from build123d import *

# Parameters (mm, degrees)
SKETCH1_R           = 14.45
BOSS_EXTRUDE1_DEPTH = 14
BOSS_EXTRUDE2_START = 7.6
SKETCH2_W           = 35.45
SKETCH2_H           = 36.25
BOSS_EXTRUDE2_DEPTH = 7.6
FILLET1_R           = 10
CUT_EXTRUDE1_REACH  = 44.204
SKETCH3_R           = 2.3
CHAMFER1_SIZE       = 0.5
CHAMFER2_SIZE       = 0.2
CHAMFER2_SIZE2      = 5.727250657
CHAMFER3_SIZE       = 0.5


with BuildPart() as part:
    # Sketch1 → Boss-Extrude1 (new body)
    with BuildSketch(Plane.XY):
        Circle(SKETCH1_R)
        with BuildLine():
            Line((-8.510102807, -10.125), (8.510102807, -10.125))
            ThreePointArc((8.510102807, -10.125), (9.652007563, -9.652007563), (10.125, -8.510102807))
            Line((10.125, -8.510102807), (10.125, 8.510102807))
            ThreePointArc((10.125, 8.510102807), (9.652007563, 9.652007563), (8.510102807, 10.125))
            Line((8.510102807, 10.125), (-8.510102807, 10.125))
            ThreePointArc((-8.510102807, 10.125), (-9.652007563, 9.652007563), (-10.125, 8.510102807))
            Line((-10.125, 8.510102807), (-10.125, -8.510102807))
            ThreePointArc((-10.125, -8.510102807), (-9.652007563, -9.652007563), (-8.510102807, -10.125))
        make_face(mode=Mode.SUBTRACT)
    extrude(amount=BOSS_EXTRUDE1_DEPTH)

    # Sketch2 → Boss-Extrude2 (add)
    with BuildSketch(Plane(origin=(0, 0, 0), x_dir=(-1, 0, 0), z_dir=(0, 0, -1)).offset(BOSS_EXTRUDE2_START)):
        with Locations((-0.4, 0)):
            Rectangle(SKETCH2_W, SKETCH2_H)
        with BuildLine():
            Line((8.510102807, -10.125), (-8.510102807, -10.125))
            ThreePointArc((-8.510102807, -10.125), (-9.652007563, -9.652007563), (-10.125, -8.510102807))
            Line((-10.125, -8.510102807), (-10.125, 8.510102807))
            ThreePointArc((-10.125, 8.510102807), (-9.652007563, 9.652007563), (-8.510102807, 10.125))
            Line((-8.510102807, 10.125), (8.510102807, 10.125))
            ThreePointArc((8.510102807, 10.125), (9.652007563, 9.652007563), (10.125, 8.510102807))
            Line((10.125, 8.510102807), (10.125, -8.510102807))
            ThreePointArc((10.125, -8.510102807), (9.652007563, -9.652007563), (8.510102807, -10.125))
        make_face(mode=Mode.SUBTRACT)
    extrude(amount=-BOSS_EXTRUDE2_DEPTH)

    # Fillet1
    fillet1_edges = [part.edges().sort_by_distance(p)[0] for p in [
        (18.125, 18.125, -3.8),
        (18.125, -18.125, -3.8),
        (-17.325, -18.125, -3.8),
        (-17.325, 18.125, -3.8),
    ]]
    fillet(fillet1_edges, radius=FILLET1_R)

    # Sketch3 → Cut-Extrude1 (cut, up to next)
    with BuildSketch(Plane.ZY.offset(17.325), mode=Mode.PRIVATE) as cut_extrude1_sk1:
        with Locations(Location((-3.8, 0, 0), (0, 0, 270))):
            Circle(SKETCH3_R)
    cut_extrude1_tool1 = extrude(cut_extrude1_sk1.sketch, amount=-CUT_EXTRUDE1_REACH, mode=Mode.PRIVATE) & part.part
    add(cut_extrude1_tool1.solids().sort_by_distance((-17.325, 0, -3.8))[0], mode=Mode.SUBTRACT)

    # Chamfer1
    chamfer1_edges = [part.edges().sort_by_distance(p)[0] for p in [
        (-9.652007563, 9.652007563, -7.6),
        (0, 10.125, -7.6),
        (9.652007563, 9.652007563, -7.6),
        (10.125, 0, -7.6),
        (9.652007563, -9.652007563, -7.6),
        (0, -10.125, -7.6),
        (-9.652007563, -9.652007563, -7.6),
        (-10.125, 0, -7.6),
        (0.4, 18.125, 0),
        (0.4, 18.125, -7.6),
        (18.125, 0, 0),
        (-17.325, 0, 0),
        (0.4, -18.125, 0),
        (-14.396067812, -15.196067812, 0),
        (15.196067812, -15.196067812, 0),
        (15.196067812, 15.196067812, 0),
        (-14.396067812, 15.196067812, 0),
        (-17.325, 0, -7.6),
        (18.125, 0, -7.6),
        (0.4, -18.125, -7.6),
        (-14.396067812, -15.196067812, -7.6),
        (15.196067812, -15.196067812, -7.6),
        (15.196067812, 15.196067812, -7.6),
        (-14.396067812, 15.196067812, -7.6),
        (-10.125, 2.3, -3.8),
        (-17.325, 2.3, -3.8),
    ]]
    chamfer(chamfer1_edges, length=CHAMFER1_SIZE)

    # Chamfer2
    chamfer2_edges = [part.edges().sort_by_distance(p)[0] for p in [
        (-14.45, 0, 0),
    ]]
    chamfer2_side = [part.faces().sort_by_distance(p)[0] for p in [
        (0.4, 17.132114111, 0),
    ]]
    chamfer(chamfer2_edges, length=CHAMFER2_SIZE, length2=CHAMFER2_SIZE2, reference=chamfer2_side[0])

    # Chamfer3
    # the kernel refuses this chamfer: 0.5 mm, written as the material it takes off along each edge
    with BuildSketch(Plane(origin=(8.510102807, -8.510102807, 14), x_dir=(0, -1, 0), z_dir=(-1, 0, 0))) as chamfer3_piece_1:
        Polygon((1.614897193 + CHAMFER3_SIZE, 0), (1.614897193, -CHAMFER3_SIZE), (1.614897193, 0), align=None)
    revolve(axis=Axis((8.510102807, -8.510102807, 14), (0, 0, 1)), revolution_arc=90, mode=Mode.SUBTRACT)
    with BuildSketch(Plane(origin=(10.125, -8.510102807, 14), x_dir=(0.9996219169112968, 2.0865614307067877e-15, 0.027495876610585647), z_dir=(0, 1, 0)), Plane(origin=(8.510102807, 10.125, 14), x_dir=(-1.877905287636107e-15, 0.9996219169112968, 0.027495876610585647), z_dir=(-1, 0, 0)), Plane(origin=(-10.125, 8.510102807, 14), x_dir=(-0.9996219169112968, 0, 0.027495876610585647), z_dir=(0, -1, 0)), Plane(origin=(-8.510102807, -10.125, 14), x_dir=(0, -0.9996219169112968, 0.027495876610585647), z_dir=(1, 0, 0))) as chamfer3_piece_2:
        Polygon((CHAMFER3_SIZE * 0.999621916911, CHAMFER3_SIZE * 0.0274958766106), (-CHAMFER3_SIZE * 0.0274958766106, CHAMFER3_SIZE * 0.999621916911), (0, 0), align=None)
    extrude(amount=17.020205615, mode=Mode.SUBTRACT)
    with BuildSketch(Plane(origin=(8.510102807, 8.510102807, 14), x_dir=(1, 0, 0), z_dir=(0, -1, 0))) as chamfer3_piece_3:
        Polygon((1.614897193 + CHAMFER3_SIZE, 0), (1.614897193, -CHAMFER3_SIZE), (1.614897193, 0), align=None)
    revolve(axis=Axis((8.510102807, 8.510102807, 14), (0, 0, 1)), revolution_arc=90, mode=Mode.SUBTRACT)
    with BuildSketch(Plane(origin=(-8.510102807, 8.510102807, 14), x_dir=(0, 1, 0), z_dir=(1, 0, 0))) as chamfer3_piece_4:
        Polygon((1.614897193 + CHAMFER3_SIZE, 0), (1.614897193, -CHAMFER3_SIZE), (1.614897193, 0), align=None)
    revolve(axis=Axis((-8.510102807, 8.510102807, 14), (0, 0, 1)), revolution_arc=90, mode=Mode.SUBTRACT)
    with BuildSketch(Plane(origin=(-8.510102807, -8.510102807, 14), x_dir=(-1, 0, 0), z_dir=(0, 1, 0))) as chamfer3_piece_5:
        Polygon((1.614897193 + CHAMFER3_SIZE, 0), (1.614897193, -CHAMFER3_SIZE), (1.614897193, 0), align=None)
    revolve(axis=Axis((-8.510102807, -8.510102807, 14), (0, 0, 1)), revolution_arc=90, mode=Mode.SUBTRACT)
    with BuildSketch(Plane(origin=(0, 0, 14), x_dir=(1, 0, 0), z_dir=(0, -1, 0))) as chamfer3_piece_6:
        Polygon((14.45, -CHAMFER3_SIZE), (14.45 - CHAMFER3_SIZE, 0), (14.45, 0), align=None)
    revolve(axis=Axis((0, 0, 14), (0, 0, 1)), mode=Mode.SUBTRACT)


solid = part.part
The model under review builds one solid part; all positions refer to its coordinate system, in mm. A direction names the side the tool comes from. Round coordinates to 2 decimals unless told otherwise and drop trailing zeros. Write each loop counter-clockwise with the first axis right and the second up, starting at its lowest first coordinate (ties: lowest second). Pieces come first, ordered by that corner, then holes. Notation, with made-up numbers: (-30, 22) - (-11, 22) arc R19 ccw to (-11, 33) - close; hole circle Ø1 at (19, 4.5). An arc over 180 degrees is marked (long way). One line per item, written item: value. Start each with the question number.
1. Consider section B-B on z = 11.5. Write out the cut boundary in (x, y) (3 decimals).
2. Consider section C-C on x = 0. Write out the cut boundary in (y, z) (3 decimals), and give its area (3 significant figures).
3. Consider section A-A on y = 0. State how many separate pieces and enclosed holes the cut face has, and give its area (3 significant figures).
4. Machinability: for faces 4 (the face through (-13.768, 0.499, -6.045)), 5 (the face through (9.734, -9.761, 13.635)), 6 (the face through (9.7, 9.6, 3.1)), 7 (the face through (9.761, 9.734, -7.235)), 8 (the face through (-11, 0, -7.6)), which of the approach directions +Z, -Z, +X, -X, +Y, -Y give a long, thin tool a straight path to every point of the face, cutting with its end or side? Answer none if there is none.
5. Clearance check with flat-ended pins moving along their axes: P1, Ø1, axis at x = -8.5, z = 1, coming from the -Y side; P2, Ø1, axis at y = 4, z = 5.5, coming from the +X side; P3, Ø1, axis at x = -9, y = -6.5, coming from the -Z side; P4, Ø5, axis at y = 3.5, z = 5.5, coming from the +X side. State where each tip first meets the part, or that it passes through.
6. To check wall thickness, follow L1, parallel to X at y = -2, z = 1.5 (3 decimals); L2, parallel to Z at x = -15.5, y = 0; L3, parallel to Z at x = -14, y = 0. State the ranges of each line that lie inside material, in increasing order. Write a range as from..to.
7. The part is to be moulded in two halves that separate along Y. For faces 1 (the face through (-12, 0, 14)), 2 (the face through (14.868, -15.018, -0.142)), 3 (the face through (0, 10.125, 3)), say which applies: released by +Y, released by -Y, zero draft, split by the parting line, or undercut.
8. Consider section D-D on z = -3.8. Write out the cut boundary in (x, y) (3 decimals).
Checks:
1. outline: circle Ø28.9 at (0, 0); hole (-10.125, -8.51) arc R1.615 ccw to (-8.51, -10.125) - (8.51, -10.125) arc R1.615 ccw to (10.125, -8.51) - (10.125, 8.51) arc R1.615 ccw to (8.51, 10.125) - (-8.51, 10.125) arc R1.615 ccw to (-10.125, 8.51) - close
2. outline: (-18.125, -7.1) - (-17.625, -7.6) - (-10.625, -7.6) - (-10.125, -7.1) - (-10.125, 13.5) - (-10.625, 14) - (-13.95, 14) - (-14.45, 13.5) - (-14.45, 5.727) - (-14.65, 0) - (-17.625, 0) - (-18.125, -0.5) - close; (10.125, -7.1) - (10.625, -7.6) - (17.625, -7.6) - (18.125, -7.1) - (18.125, -0.5) - (17.625, 0) - (14.65, 0) - (14.45, 5.727) - (14.45, 13.5) - (13.95, 14) - (10.625, 14) - (10.125, 13.5) - close
2. area: 243 mm^2
3. separate pieces: 3
3. enclosed holes: 0
3. area: 203 mm^2
4. face 4: -X
4. face 5: +Z
4. face 6: +Z, -Z
4. face 7: -Z
4. face 8: -Z, +X, -X, +Y, -Y
5. P1: stops at y = -12.23
5. P2: stops at x = 14.03
5. P3: passes through
5. P4: stops at x = 14.44
6. L1: x = -14.46..-10.125, 10.125..14.46
6. L2: z = -7.6..-6.1, -1.5..0
6. L3: z = -7.6..-6.1, -1.5..13.95
7. face 1: zero draft
7. face 2: released by -Y
7. face 3: undercut
8. outline: (-17.325, -8.125) arc R10 ccw to (-7.325, -18.125) - (8.125, -18.125) arc R10 ccw to (18.125, -8.125) - (18.125, 8.125) arc R10 ccw to (8.125, 18.125) - (-7.325, 18.125) arc R10 ccw to (-17.325, 8.125) - (-17.325, 2.8) - (-16.825, 2.3) - (-10.625, 2.3) - (-10.125, 2.8) - (-10.125, 8.51) arc R1.615 cw to (-8.51, 10.125) - (8.51, 10.125) arc R1.615 cw to (10.125, 8.51) - (10.125, -8.51) arc R1.615 cw to (8.51, -10.125) - (-8.51, -10.125) arc R1.615 cw to (-10.125, -8.51) - (-10.125, -2.8) - (-10.625, -2.3) - (-16.825, -2.3) - (-17.325, -2.8) - close
